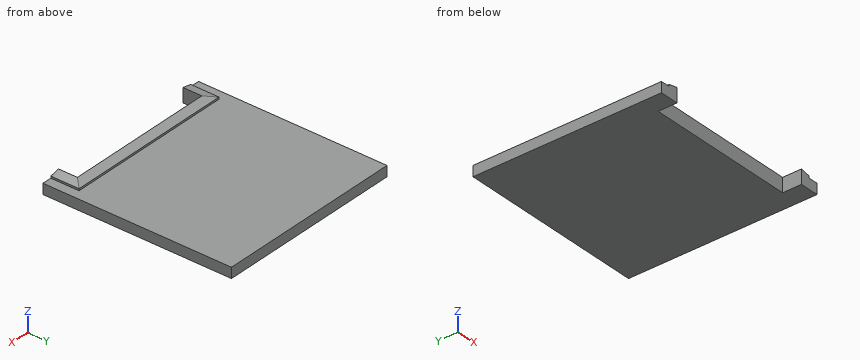
Autodesk Inventor part; units mm, degrees
ref_plane "Work Plane1" through (0, 0, 1.651) normal (0, 0, 1) x (1, 0, 0)
ref_plane "YZ Plane" through (0, 0, 0) normal (1, 0, 0) x (0, 1, 0)
ref_plane "XZ Plane" through (0, 0, 0) normal (0, 1, 0) x (-1, 0, 0)
sketch "Sketch1" plane through (0, 0, 0) normal (0, 0, 1) x (1, 0, 0)
  line L0 (-12.7, 38.1) -> (12.7, 38.1)
  line L1 (12.7, 38.1) -> (12.7, -38.1)
  line L2 (12.7, -38.1) -> (-12.7, -38.1)
  line L3 (-12.7, -38.1) -> (-12.7, 38.1)
  line L4 (-12.7, 38.1) -> (12.7, -38.1) construction
  line L5 (12.7, 38.1) -> (-12.7, -38.1) construction
  point P0 (0, 0)
  dimension "d0" = 25.4
  dimension "d1" = 76.2
extrude "Extrusion1" add sketch "Sketch1" along normal blind 1.397
sketch "Sketch2" plane through (0, 0, 1.397) normal (0, 0, 1) x (1, 0, 0)
  line L0 (-10.16, -38.1) -> (10.16, -38.1)
  line L1 (10.16, -38.1) -> (10.16, 15.24)
  line L2 (10.16, 15.24) -> (-10.16, 15.24)
  line L3 (-10.16, 15.24) -> (-10.16, -38.1)
  line L4 (-12.7, -38.1) -> (12.7, -38.1)
  point P0 (0, 0)
  point P1 (0, -38.1)
  dimension "d4" = 20.32
  dimension "d5" = 53.34
extrude "Extrusion2" cut sketch "Sketch2" against normal through all
sketch "Sketch3" plane through (12.7, -38.1, 0) normal (1, 0, 0) x (0, 0, -1)
  line L0 (0, 76.2) -> (0, 0)
  line L1 (0, 76.2) -> (-1.397, 76.2)
  line L2 (-1.397, 0) -> (-1.397, 76.2)
  line L3 (0, 0) -> (-1.397, 0)
  line L4 (-1.397, 0) -> (-1.905, 0)
  line L5 (-1.397, 0) -> (-1.397, 1.27)
  line L6 (-1.397, 53.34) -> (-1.397, 0)
  line L7 (-1.651, 1.27) -> (-1.397, 1.27)
  line L8 (-1.651, 1.27) -> (-1.905, 0)
  point P0 (0, 38.1)
  dimension "d8" = 0.508
  dimension "d9" = 1.27
  dimension "d10" = 0.254
ref_plane "Work Plane1" through (0, 0, 1.651) normal (0, 0, 1) x (1, 0, 0)
sketch "Sketch6" plane through (0, 0, 1.651) normal (0, 0, 1) x (1, 0, 0)
  line L0 (12.7, -36.83) -> (12.7, -38.1)
  line L1 (12.7, -38.1) -> (12.7, 38.1)
  line L2 (12.7, -37.465) -> (10.795, -37.465)
  line L3 (10.16, -38.1) -> (12.7, -38.1)
  line L4 (10.16, 15.24) -> (10.16, -38.1)
  line L5 (10.795, -37.465) -> (10.795, 15.875)
  line L6 (10.795, 15.875) -> (-10.795, 15.875)
  line L7 (-10.795, 15.875) -> (-10.795, -37.465)
  line L8 (-10.795, -37.465) -> (-12.7255, -37.465)
  line L9 (-12.7, -38.1) -> (-10.16, -38.1)
  line L10 (-10.16, -38.1) -> (-10.16, 15.24)
  line L11 (-10.16, 15.24) -> (10.16, 15.24)
  point P0 (0, 0)
  dimension "d12" = 0.635
  dimension "d13" = 0.635
  dimension "d14" = 0.635
  dimension "d15" = 0.635
  dimension "d16" = 0.635
sweep "Sweep1" add profiles "Sketch3" path "Sketch6" path curves L2 L5 L6 L7 L8 contours L4 L8 L7 L2
ref_plane "Work Plane3" through (-12.7, 12.7, 0) normal (0, -1, 0) x (1, 0, 0)
ref_plane "Work Plane2" through (-12.7, -12.7, 0) normal (0, -1, 0) x (1, 0, 0)
split "Split3" plane through (-12.7, -12.7, 0) removes the side toward (0, -1, 0)
split "Split5" plane through (-12.7, 12.7, 0) removes the side toward (0, -1, 0)
properties part number "door-frame"
The model under review builds one solid part; all positions refer to its coordinate system, in mm. Give positions to 0.01 mm unless a question says otherwise; leave off trailing zeros. Order: outer loops, then holes, each group sorted by start corner. A loop starts at its lowest first (then second) coordinate and runs counter-clockwise, first axis right, second up. Notation, with made-up numbers: M 51,-1 L 94,-1 A13 cw 94,22 Z; hole C 41.25,21.5 d3. An arc over 180 degrees is marked long. Use one line per item in the form item = value. Start each with the question number.
Item 1: We need section B-B on z = 1. Give the boundary of the cut face in (x, y), plus the area to 3 significant figures.
Item 2: We need section A-A on x = 2. Give the boundary of the cut face in (y, z) (3 decimals).
Item 3: We need section C-C on y = 17.75. Give the boundary of the cut face in (x, z).
Item 4: To check wall thickness, follow line 1 along X through (y, z) = (14.75, 1.35); line 2 along Z through (x, y) = (5.5, 25.25); line 3 along Y through (x, z) = (6, 1.35). State the ranges of each line that lie inside material, in increasing order. Write a range as from..to.
Item 5: Insertion check: pin 1 Ø12.5 at (x, y) = (-1, 30) entering from +Z. The pin has a flat end and moves straight along its axis. Give the tip position at first contact, or say it passes through.
Completed:
q1.outline = M -12.7,12.7 L -10.16,12.7 L -10.16,15.24 L 10.16,15.24 L 10.16,12.7 L 12.7,12.7 L 12.7,38.1 L -12.7,38.1 Z
q1.area = 594 mm²
q2.outline = M 15.24,0 L 38.1,0 L 38.1,1.397 L 16.51,1.397 L 16.51,1.651 L 15.24,1.905 Z
q3.outline = M -12.7,0 L 12.7,0 L 12.7,1.4 L -12.7,1.4 Z
q4.line_1 = -12.7..-10.16, 10.16..12.7
q4.line_2 = 0..1.4
q4.line_3 = 15.24..38.1
q5.pin_1 = 1.4
